Model file for the job. Use its own axes, mm. A direction names the side the tool comes from. Round coordinates to 2 decimals unless told otherwise and drop trailing zeros. Loops run counter-clockwise (first coordinate to the right, second up) from the corner with the lowest first, then second, coordinate; pieces in that order, holes last. Notation, with made-up numbers: (-14, 78.5) - (26, 78.5) arc R30 cw to (26, 111.5) - close; hole circle Ø3 at (15.25, -13.5). An arc over 180 degrees is marked (long way). Answer as a JSON object with one key per item and string values.
Autodesk Inventor part; units mm, degrees
ref_plane "Work Plane1" through (0, 0, -15) normal (0, 0, 1) x (1, 0, 0)
ref_plane "YZ Plane" through (0, 0, 0) normal (1, 0, 0) x (0, 1, 0)
ref_plane "XZ Plane" through (0, 0, 0) normal (0, 1, 0) x (-1, 0, 0)
sketch "Sketch1" plane through (0, 0, 0) normal (0, 0, 1) x (1, 0, 0)
  line L0 (0, 0) -> (25, 0)
  line L1 (25, 0) -> (25, 40)
  line L2 (25, 40) -> (0, 40)
  line L3 (0, 40) -> (0, 0)
  dimension "d1" = 25
  dimension "d2" = 40
  dimension "d3" = 25
extrude "Extrusion1" add sketch "Sketch1" against normal blind 30
sketch "Sketch2" plane through (25, 0, 0) normal (1, 0, 0) x (0, 0, -1)
  line L0 (0, 0) -> (30, 0)
  circle A0 centre (15, 6.56) radius 2.46
extrude "Extrusion2" cut sketch "Sketch2" against normal blind 30
sketch "Sketch3" plane through (0, 0, 0) normal (-1, 0, 0) x (0, 0, 1)
  line L0 (0, 0) -> (-30, 0)
  line L1 (-25.05, 0) -> (-4.95, 0)
  line L2 (-4.95, 0) -> (-4.95, 33.12)
  line L3 (-4.95, 33.12) -> (-25.05, 33.12)
  line L4 (-25.05, 33.12) -> (-25.05, 0)
  dimension "d11" = 20.1
extrude "Extrusion3" cut sketch "Sketch3" against normal blind 20
sketch "Sketch4" plane through (0, 0, 0) normal (0, -1, 0) x (1, 0, 0)
  line L0 (20, -4.95) -> (20, -25.05)
  line L1 (20, -15) -> (25, -15)
  line L2 (25, 0) -> (25, -30)
  line L3 (20, -8.025) -> (25, -8.025)
  line L4 (25, -8.025) -> (25, -21.975)
  line L5 (25, -21.975) -> (20, -21.975)
  line L6 (20, -21.975) -> (20, -8.025)
  line L7 (20, -8.025) -> (25, -21.975) construction
  line L8 (25, -8.025) -> (20, -21.975) construction
  line L9 (25, -12.54) -> (25, -17.46)
  point P0 (0, 0)
  point P1 (22.5, -15)
  dimension "d14" = 13.95
extrude "Extrusion4" add sketch "Sketch4" along normal blind 15
sketch "Sketch5" plane through (20, 0, 0) normal (-1, 0, 0) x (0, 0, 1)
  circle A0 centre (-15, 6.56) radius 2.46
  circle A1 centre (-15, 6.56) radius 4.7025
  circle A2 centre (-15, 6.56) radius 2.46
  circle A3 centre (-15, 6.56) radius 2.46
  point P0 (0, 0)
  dimension "d17" = 9.405
extrude "Extrusion5" cut sketch "Sketch5" against normal blind 2.1
sketch "Sketch6" plane through (25, 0, 0) normal (1, 0, 0) x (0, 0, -1)
  circle A0 centre (15, 6.56) radius 4.7025
  line L0 (15, 6.56) -> (15, 23.56)
  circle A1 centre (15, 23.56) radius 2.46
  point P0 (0, 0)
  dimension "d20" = 17
  dimension "d21" = 4.92
extrude "Extrusion6" cut sketch "Sketch6" against normal blind 10 contours A1
sketch "Sketch7" plane through (20, 0, 0) normal (-1, 0, 0) x (0, 0, 1)
  circle A0 centre (-15, 23.56) radius 2.46
  circle A1 centre (-15, 23.56) radius 4.7025
  point P0 (0, 0)
  dimension "d24" = 9.405
extrude "Extrusion7" cut sketch "Sketch7" against normal blind 2.1
sketch "Sketch9" plane through (25, 0, 0) normal (1, 0, 0) x (0, 0, -1)
  circle A0 centre (15, 6.56) radius 2.46
  circle A1 centre (15, 6.56) radius 2.46
  circle A2 centre (15, 23.56) radius 2.46
  circle A3 centre (15, 23.56) radius 2.46
  line L0 (30, 40) -> (30, 0)
  line L1 (30, 0) -> (30, 40)
  line L2 (30, 40) -> (0, 40)
  line L3 (0, 40) -> (0, 0)
  line L4 (0, 0) -> (8.025, 0)
  line L5 (21.975, 0) -> (21.975, -15)
  line L6 (21.975, -15) -> (8.025, -15)
  line L7 (8.025, -15) -> (8.025, 0)
  line L8 (0, 0) -> (8.025, 0)
  line L9 (21.975, 0) -> (30, 0)
extrude "Extrusion8" add sketch "Sketch9" along normal blind 5
sketch "Sketch10" plane through (0, 40, 0) normal (0, 1, 0) x (1, 0, 0)
  line L0 (0, 30) -> (30, 30)
  line L1 (30, 0) -> (0, 0)
  line L2 (0, 30) -> (30, 30)
  line L3 (30, 30) -> (30, 0)
  line L4 (30, 0) -> (0, 0)
  line L5 (0, 0) -> (0, 30)
extrude "Extrusion9" add sketch "Sketch10" along normal blind 30
sketch "Sketch12" plane through (30, 0, 0) normal (1, 0, 0) x (0, 0, -1)
  circle A0 centre (15, 6.56) radius 2.46
  line L0 (15, 6.56) -> (15, 15.06)
  circle A1 centre (15, 15.06) radius 2.525
  point P0 (0, 0)
  dimension "d31" = 8.5
  dimension "d33" = 5.05
extrude "Extrusion10" cut sketch "Sketch12" against normal blind 30 contours A1
sketch "Sketch14" plane through (0, 0, 0) normal (0, 0, 1) x (1, 0, 0)
  line L0 (30, 70) -> (0, 70)
  line L1 (0, 70) -> (0, 85)
  line L2 (30, 0) -> (30, 70)
  line L3 (30, 109) -> (30, 70)
  line L4 (30, 105) -> (30, 100)
  line L5 (-12, 124) -> (15, 124)
  line L6 (-8, 122) -> (-12, 124)
  line L7 (-8, 122) -> (-4, 112)
  line L8 (-8, 102) -> (-12, 100)
  line L9 (-8, 102) -> (-4, 112)
  line L10 (30, 109) -> (15, 124)
  line L11 (0, 85) -> (0, 100)
  line L12 (0, 100) -> (-12, 100)
  point P0 (0, 0)
  dimension "d69" = 12
extrude "Extrusion12" add sketch "Sketch14" against normal blind 30
sketch "Sketch15" plane through (0, 0, -25.05) normal (-1, 0, 0) x (0, 0, 1)
  line L0 (0, 33.12) -> (20.1, 33.12)
  line L1 (20.1, 33.12) -> (20.1, 0)
  line L2 (0, 33.12) -> (20.1, 33.12)
  line L3 (20.1, 33.12) -> (20.1, 31.1)
  line L4 (20.1, 31.1) -> (0, 31.1)
  line L5 (0, 31.1) -> (0, 33.12)
  point P0 (25.05, 0)
  dimension "d57" = 2.02
extrude "Extrusion13" add sketch "Sketch15" against normal blind 20
sketch "Sketch19" plane through (0, 0, 0) normal (0, 0, 1) x (1, 0, 0)
  line L0 (0, 100) -> (-12, 100)
  line L1 (0, 100) -> (-12, 100)
  line L2 (-12, 100) -> (-8, 102)
  line L3 (-12, 100) -> (-8, 102)
  line L4 (-8, 102) -> (-4, 112)
  line L5 (-8, 102) -> (-4, 112)
  line L6 (-4, 112) -> (-8, 122)
  line L7 (-4, 112) -> (-8, 122)
  line L8 (-8, 122) -> (-12, 124)
  line L9 (-8, 122) -> (-12, 124)
  line L10 (-12, 124) -> (15, 124)
  line L11 (-12, 124) -> (15, 124)
  line L12 (15, 124) -> (30, 109)
  line L13 (15, 124) -> (30, 109)
  line L14 (30, 109) -> (30, 89)
  line L15 (30, 89) -> (0, 89)
  line L16 (0, 89) -> (0, 100)
  point P0 (0, 0)
  dimension "d71" = 20
  dimension "d72" = 30
extrude "Extrusion14" add sketch "Sketch19" along normal blind 45
ref_plane "Work Plane1" through (0, 0, -15) normal (0, 0, 1) x (1, 0, 0)
mirror "Mirror1" about plane through (0, 0, -15) normal (0, 0, 1) of "Extrusion14"
properties part number "rec_b_20mm_x_120mm"
1) Slice it at D-D on z = -38. List the corners of the cut face in (x, y).
Values follow:
{"outline": "(-12, 100) - (0, 100) - (0, 89) - (30, 89) - (30, 109) - (15, 124) - (-12, 124) - (-8, 122) - (-4, 112) - (-8, 102) - close"}
2) Two-plate mould, pull along Z, no slides. Class faces 6 (the flat face through (15, 45, -30)), 7 (the flat face through (23, 116, -14)), 8 (the cylindrical face through (21.035, 7.973, -10.515)): pulls with the +Z half, pulls with the -Z half, needs draft (parallel to the pull), parting line crosses it, or undercut.
Values follow:
{"face 6": "pulls with the -Z half", "face 7": "needs draft", "face 8": "undercut"}
3) Slice it at B-B on z = -15. Count the separate pieces of the cut face and the enclosed holes in it, then the cut area to 3 significant figures.
Values follow:
{"separate pieces": "4", "enclosed holes": "0", "area": "3,130 mm²"}
4) Drop flat-ended pins along their axis: P1, Ø6, axis at x = -6.5, z = -35, coming from the -Y side; P2, Ø15, axis at x = 17, z = 20.5, coming from the -Y side; P3, Ø3, axis at x = 26.5, y = -7, coming from the +Z side (3 decimals); P4, Ø16, axis at x = 15, z = -16.5, coming from the -Y side. Give the stop position or say it passes through.
Values follow:
{"P1": "y = 100", "P2": "y = 89", "P3": "z = -8.025", "P4": "y = -15"}
5) Probe probe 1 along Y at (x, z) = (22.5, -15) (3 decimals); probe 2 along Z at (x, y) = (21, 6); probe 3 along Z at (x, y) = (2, 84.5). List the from-to ranges inside material, lowest first.
Values follow:
{"probe 1": "-15 to 4.1, 9.02 to 12.535, 17.585 to 21.1, 26.02 to 116.5", "probe 2": "-30 to -19.67, -10.33 to 0", "probe 3": "-30 to 0"}
6) Slice it at C-C on x = 18. List the corners of the cut face in (y, z), then the cut area to 3 significant figures.
Values follow:
{"outline": "(0, -30) - (89, -30) - (89, -75) - (121, -75) - (121, 45) - (89, 45) - (89, 0) - (0, 0) - (0, -4.95) - (31.1, -4.95) - (31.1, -25.05) - (0, -25.05) - close", "area": "5,880 mm²"}
7) Slice it at A-A on y = 15.06. List the corners of the cut face in (x, z) (3 decimals).
Values follow:
{"outline": "(0, -30) - (30, -30) - (30, -17.525) - (20, -17.525) - (20, -25.05) - (0, -25.05) - close; (0, -4.95) - (20, -4.95) - (20, -12.475) - (30, -12.475) - (30, 0) - (0, 0) - close"}
8) Tool access for faces 1 (the flat face through (15, 89, -52)), 2 (the flat face through (-6, 107, -14)), 3 (the flat face through (25, -8, -8.025)), 4 (the flat face through (-6, 100, -14)), 5 (the flat face through (20, 8, -20)): list every direction of +Z, -Z, +X, -X, +Y, -Y with a clear straight run to the whole face (end or side of a thin tool).
Values follow:
{"face 1": "-Z, +X, -X, -Y", "face 2": "+Z, -Z, -X", "face 3": "+Z, +X, -X, -Y", "face 4": "+Z, -Z, -X, -Y", "face 5": "-X, -Y"}
